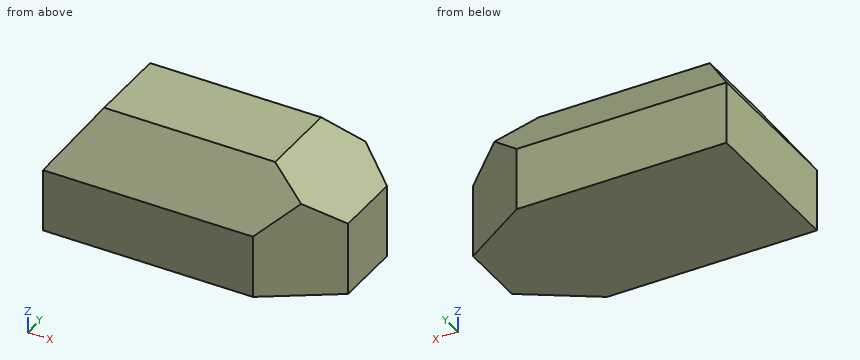
```python
from build123d import *

# Parameters (mm, degrees)
F0_W       = 10.2235
F0_H       = 5.7912
F1_DEPTH   = 4.3307
F2_SIZE2   = 1.4228217176
F2_SIZE    = 2.032
F3_SIZE2   = 1.6494952867
F3_SIZE    = 2.54
F3_2_SIZE2 = 1.6494952867
F3_2_SIZE  = 2.54
F3_3_SIZE2 = 1.6494952867
F3_3_SIZE  = 2.54


with BuildPart() as f1:
    # F0 (on Top) → F1 (new body)
    with BuildSketch(Plane.XY):
        Rectangle(F0_W, F0_H)
    extrude(amount=F1_DEPTH)

    # F2
    f2_edges = [f1.edges().sort_by_distance(p)[0] for p in [
        (0, -2.8956, 4.3307),
        (0, 2.8956, 4.3307),
        (-5.11175, 0, 4.3307),
    ]]
    chamfer(f2_edges, length=F2_SIZE, length2=F2_SIZE2)

    # F3
    f3_edges = [f1.edges().sort_by_distance(p)[0] for p in [
        (5.11175, 0, 4.3307),
    ]]
    f3_side = f1.faces().sort_by_distance((0.711411, 0, 4.3307))[0]
    chamfer(f3_edges, length=F3_SIZE, length2=F3_SIZE2, reference=f3_side)

    # F3#2
    f3_2_edges = [f1.edges().sort_by_distance(p)[0] for p in [
        (5.11175, -2.8956, 1.14935),
    ]]
    f3_2_side = f1.faces().sort_by_distance((0, -2.8956, 1.14935))[0]
    chamfer(f3_2_edges, length=F3_2_SIZE, length2=F3_2_SIZE2, reference=f3_2_side)

    # F3#3
    f3_3_edges = [f1.edges().sort_by_distance(p)[0] for p in [
        (5.11175, 2.8956, 1.14935),
    ]]
    f3_3_side = f1.faces().sort_by_distance((0, 2.8956, 1.14935))[0]
    chamfer(f3_3_edges, length=F3_3_SIZE, length2=F3_3_SIZE2, reference=f3_3_side)


solid = f1.part
```
Read the model definition and answer for the solid it produces. Units are mm, in the model's axes. Coordinates: 2 decimals unless noted, no trailing zeros. Loops run counter-clockwise (first coordinate to the right, second up) from the corner with the lowest first, then second, coordinate; pieces in that order, holes last.
(1) Consider line 1 along X through (y, z) = (-0.05, 3.4); line 2 along X through (y, z) = (2.15, 1.25); line 3 along Z through (x, y) = (2.25, -1.55). Determine where each line is inside the solid, lowest interval first.
Solution:
line 1: x = -4.34 to 4
line 2: x = -5.11 to 3.72
line 3: z = 0 to 4.22
(2) The part is cut by section C-C (y = -2.45). Determine the outline of the cut face in (x, z).
Solution:
outline: (-5.11, 0) - (3.26, 0) - (3.26, 2.94) - (-4.67, 2.94) - (-5.11, 2.3) - close
(3) The part is cut by section B-B (x = 1.5). Determine the outline of the cut face in (y, z).
Solution:
outline: (-2.9, 0) - (2.9, 0) - (2.9, 2.3) - (1.47, 4.33) - (-1.47, 4.33) - (-2.9, 2.3) - close
(4) The part is cut by section A-A (y = -0.85). Determine the outline of the cut face in (x, z).
Solution:
outline: (-5.11, 0) - (5.11, 0) - (5.11, 2.68) - (2.57, 4.33) - (-3.69, 4.33) - (-5.11, 2.3) - close
(5) The part is cut by section D-D (x = 4.25). Determine the outline of the cut face in (y, z).
Solution:
outline: (-1.81, 0) - (1.81, 0) - (1.81, 3.24) - (-1.81, 3.24) - close
